Geometry check sheet. Reference: the model listing, model coordinates, mm. A direction names the side the tool comes from. Round coordinates to 2 decimals unless told otherwise and drop trailing zeros. Write each loop counter-clockwise with the first axis right and the second up, starting at its lowest first coordinate (ties: lowest second). Pieces come first, ordered by that corner, then holes.
from build123d import *

# Parameters (mm, degrees)
SKETCH_W        = 24.2
SKETCH_H        = 24
PAD_DEPTH       = 2.7
SKETCH001_W     = 24.2
SKETCH001_H     = 3
PAD001_DEPTH    = 20
POCKET_DEPTH    = 1.5
CHAMFER_SIZE    = 3
SKETCH003_W     = 17
SKETCH003_H     = 3
POCKET001_DEPTH = 21.001
SKETCH004_W     = 17
SKETCH004_H     = 1
POCKET002_DEPTH = 6
SKETCH005_R     = 4.9
POCKET003_DEPTH = 2.3
SKETCH006_R     = 6.2
POCKET004_DEPTH = 0.7
SKETCH007_R     = 1.6
PAD002_DEPTH    = 2.7
FILLET_R        = 2


with BuildPart() as part:
    # Sketch → Pad (new body)
    with BuildSketch(Plane.XY):
        Rectangle(SKETCH_W, SKETCH_H)
        with BuildLine():
            ThreePointArc((-10.5, 4.7), (-11.6, 3.6), (-10.5, 2.5))
            Line((-10.5, 2.5), (-8.5, 2.5))
            ThreePointArc((-8.5, 2.5), (-7.4, 3.6), (-8.5, 4.7))
            Line((-8.5, 4.7), (-10.5, 4.7))
        make_face(mode=Mode.SUBTRACT)
        with BuildLine():
            ThreePointArc((-10.5, -8.8), (-11.6, -9.9), (-10.5, -11))
            Line((-10.5, -11), (-8.5, -11))
            ThreePointArc((-8.5, -11), (-7.4, -9.9), (-8.5, -8.8))
            Line((-8.5, -8.8), (-10.5, -8.8))
        make_face(mode=Mode.SUBTRACT)
        with BuildLine():
            ThreePointArc((10.5, -11), (11.6, -9.9), (10.5, -8.8))
            Line((10.5, -8.8), (8.5, -8.8))
            ThreePointArc((8.5, -8.8), (7.4, -9.9), (8.5, -11))
            Line((8.5, -11), (10.5, -11))
        make_face(mode=Mode.SUBTRACT)
        with BuildLine():
            ThreePointArc((10.5, 2.5), (11.6, 3.6), (10.5, 4.7))
            Line((10.5, 4.7), (8.5, 4.7))
            ThreePointArc((8.5, 4.7), (7.4, 3.6), (8.5, 2.5))
            Line((8.5, 2.5), (10.5, 2.5))
        make_face(mode=Mode.SUBTRACT)
    extrude(amount=PAD_DEPTH)

    # Sketch001 (on Face21 of Pad) → Pad001 (join)
    with BuildSketch(Plane(origin=(0, 0, 0), x_dir=(1, 0, 0), z_dir=(0, 0, -1))):
        with Locations((0, -10.5)):
            Rectangle(SKETCH001_W, SKETCH001_H)
    extrude(amount=PAD001_DEPTH)

    # Sketch002 (on Face5 of Pad001) → Pocket (cut)
    with BuildSketch(Plane.XY.offset(2.7)):
        with BuildLine():
            ThreePointArc((-7, 0.35), (-10.5, -3.15), (-7, -6.65))
            Line((-7, -6.65), (7, -6.65))
            ThreePointArc((7, -6.65), (10.5, -3.15), (7, 0.35))
            Line((7, 0.35), (-7, 0.35))
        make_face()
    extrude(amount=-POCKET_DEPTH, mode=Mode.SUBTRACT)

    # Chamfer
    chamfer_edges = [part.edges().sort_by_distance(p)[0] for p in [
        (0, 9, 0),
    ]]
    chamfer(chamfer_edges, length=CHAMFER_SIZE)

    # Sketch003 (on Face25 of Chamfer) → Pocket001 (cut, through all)
    with BuildSketch(Plane.XZ.offset(-9)):
        with Locations((0, -1.5)):
            Rectangle(SKETCH003_W, SKETCH003_H)
    extrude(amount=POCKET001_DEPTH, mode=Mode.SUBTRACT)

    # Sketch004 (on Face6 of Pocket001) → Pocket002 (cut)
    with BuildSketch(Plane(origin=(0, 12, 0), x_dir=(-1, 0, 0), z_dir=(0, 1, 0))):
        Rectangle(SKETCH004_W, SKETCH004_H)
    extrude(amount=-POCKET002_DEPTH, mode=Mode.SUBTRACT)

    # Sketch005 (on Face17 of Pocket002) → Pocket003 (cut)
    with BuildSketch(Plane(origin=(0, 12, 0), x_dir=(-1, 0, 0), z_dir=(0, 1, 0))):
        with Locations((0, -10)):
            Circle(SKETCH005_R)
    extrude(amount=-POCKET003_DEPTH, mode=Mode.SUBTRACT)

    # Sketch006 (on Face15 of Pocket003) → Pocket004 (cut)
    with BuildSketch(Plane.XZ.offset(-9)):
        with Locations((0, -10)):
            Circle(SKETCH006_R)
    extrude(amount=-POCKET004_DEPTH, mode=Mode.SUBTRACT)

    # Sketch007 (on Face5 of Pocket004) → Pad002 (join)
    with BuildSketch(Plane.XY.offset(2.7)):
        with BuildLine():
            ThreePointArc((-19.442827, 2.508799), (-20.3, 0), (-19.442827, -2.508799))
            Line((-12.1, -12), (-19.442827, -2.508799))
            Line((-12.1, -12), (-12.1, 12))
            Line((-12.1, 12), (-19.442827, 2.508799))
        make_face()
        with Locations((-16.2, 0)):
            Circle(SKETCH007_R, mode=Mode.SUBTRACT)
        with BuildLine():
            ThreePointArc((19.442827, -2.508799), (20.3, 0), (19.442827, 2.508799))
            Line((12.1, 12), (19.442827, 2.508799))
            Line((12.1, 12), (12.1, -12))
            Line((12.1, -12), (19.442827, -2.508799))
        make_face()
        with Locations((16.2, 0)):
            Circle(SKETCH007_R, mode=Mode.SUBTRACT)
    extrude(amount=-PAD002_DEPTH)

    # Fillet
    fillet_edges = [part.edges().sort_by_distance(p)[0] for p in [
        (12.1, -12, 1.35),
        (-12.1, -12, 1.35),
        (12.1, 10.5, -20),
        (-12.1, 10.5, -20),
    ]]
    fillet(fillet_edges, radius=FILLET_R)


solid = part.part
1. Depth check by flat-ended pin: pin 1 Ø8 at (x, y) = (-8, 0.5) entering from -Z; pin 2 Ø11.5 at (x, z) = (0, -10) entering from +Y; pin 3 Ø3.5 at (x, y) = (0.5, -4) entering from +Z; pin 4 Ø2 at (x, z) = (-9.5, -8.5) entering from -Y. Enter the tip coordinate at first touch or a pass-through.
2. Section check A-A (z = -10). Record the cut outline in (x, y), plus the area to 3 significant figures.
3. Section check B-B (x = -2). Record the cut outline in (y, z), plus the area to 3 significant figures.
4. Section check C-C (y = 3.6). Record the cut outline in (x, z).
5. Section check D-D (x = -17). Record the cut outline in (y, z), plus the area to 3 significant figures.
6. Release check for a two-part mould opening along Y. For faces 1 (the face through (-15.72, 7.32, 1.37)), 2 (the face through (-9, -8.8, 1)), 3 (the face through (0, 3, 2.7)) record: +Y half, -Y half, draft (parallel to the pull), parting line (faces both ways), or undercut.
7. Access from +Z, -Z, +X, -X, +Y, -Y to the whole of each face (thin tool, end or side, straight path). Record for faces 4 (the face through (-12.1, 10, -9)), 5 (the face through (-7.4, -9.9, 1.3)), 6 (the face through (0, 9, -17)).
8. Scan lines: line 1 along Z through (x, y) = (0, 9.2); line 2 along Z through (x, y) = (0, 10.8); line 3 along Z through (x, y) = (-7, 9.75). Record each from-to range of solid material in increasing order.
Results below:
1. pin 1: stops at z = 0
1. pin 2: stops at y = 12
1. pin 3: stops at z = 1.2
1. pin 4: stops at y = 9
2. outline: (-12.1, 9) - (-6.2, 9) - (-6.2, 9.7) - (-4.9, 9.7) - (-4.9, 12) - (-12.1, 12) - close; (4.9, 9.7) - (6.2, 9.7) - (6.2, 9) - (12.1, 9) - (12.1, 12) - (4.9, 12) - close
2. area: 41.4 mm2
3. outline: (-12, 0) - (6, 0) - (6, 0.5) - (12, 0.5) - (12, 2.7) - (0.35, 2.7) - (0.35, 1.2) - (-6.65, 1.2) - (-6.65, 2.7) - (-12, 2.7) - close; (9, -20) - (12, -20) - (12, -14.47) - (9.7, -14.47) - (9.7, -15.87) - (9, -15.87) - close; (9, -4.13) - (9.7, -4.13) - (9.7, -5.53) - (12, -5.53) - (12, -0.5) - (9, -0.5) - close
3. area: 81.0 mm2
4. outline: (-18.6, 0) - (-11.6, 0) - (-11.6, 2.7) - (-18.6, 2.7) - close; (-7.4, 0) - (7.4, 0) - (7.4, 2.7) - (-7.4, 2.7) - close; (11.6, 0) - (18.6, 0) - (18.6, 2.7) - (11.6, 2.7) - close
5. outline: (-5.67, 0) - (-1.39, 0) - (-1.39, 2.7) - (-5.67, 2.7) - close; (1.39, 0) - (5.67, 0) - (5.67, 2.7) - (1.39, 2.7) - close
5. area: 23.1 mm2
6. face 1: +Y half
6. face 2: undercut
6. face 3: draft
7. face 4: -Z, -X, +Y, -Y
7. face 5: +Z, -Z
7. face 6: -Z, -Y
8. line 1: z = -20 to -16.2, -3.8 to -0.5, 0.5 to 2.7
8. line 2: z = -20 to -14.9, -5.1 to -0.5, 0.5 to 2.7
8. line 3: z = -20 to -0.5, 0.5 to 2.7
